```python
from build123d import *

# Parameters (mm, degrees)
CROQUIS1_W                 = 15
CROQUIS1_H                 = 13
SALIENTE_EXTRUIR1_DEPTH    = 3
REDONDEO1_R                = 3
CROQUIS6_R                 = 3
SALIENTE_EXTRUIR2_DEPTH    = 6
CORTAR_EXTRUIR1_DEPTH      = 66.261014396
CORTAR_EXTRUIR1_DEPTH_BACK = 66.261014396
CROQUIS2_R                 = 1.75
CORTAR_EXTRUIR2_DEPTH      = 63.24949799
CORTAR_EXTRUIR2_DEPTH_BACK = 63.24949799
CROQUIS3_R                 = 1.75
REDONDEO2_R                = 3


with BuildPart() as part:
    # Croquis1 → Saliente-Extruir1 (new, symmetric)
    with BuildSketch(Plane(origin=(0, 0, 0), x_dir=(1, 0, 0), z_dir=(0, 1, 0))):
        Polygon((0, 0), (0, 8), (14, 8), (14, 21), (0, 21), (0, 29), (55, 29), (55, 21), (41, 21), (41, 8), (55, 8), (55, 0), align=None)
        with Locations((27.5, 14.5)):
            Rectangle(CROQUIS1_W, CROQUIS1_H, mode=Mode.SUBTRACT)
    extrude(amount=SALIENTE_EXTRUIR1_DEPTH, both=True)

    # Redondeo1
    redondeo1_edges = [part.edges().sort_by_distance(p)[0] for p in [
        (0, -3, -4),
        (0, 3, -4),
        (0, -3, -25),
        (0, 3, -25),
        (55, -3, -4),
        (55, 3, -4),
        (55, 3, -25),
        (55, -3, -25),
    ]]
    fillet(redondeo1_edges, radius=REDONDEO1_R - 0.0001)  # a hair under: the kernel refuses the full size

    # Croquis6 → Saliente-Extruir2 (add)
    with BuildSketch(Plane.XY):
        with Locations(Location((3, 0, 0), (0, 0, 180))):
            Circle(CROQUIS6_R)
    extrude(amount=SALIENTE_EXTRUIR2_DEPTH)

    # Croquis2 → Cortar-Extruir1 (cut, two sides: drawn at the far end of the back side and taken through both)
    with BuildSketch(Plane.XY.offset(6).offset(-CORTAR_EXTRUIR1_DEPTH_BACK)):
        with Locations((3, 0)):
            Circle(CROQUIS2_R)
    extrude(amount=CORTAR_EXTRUIR1_DEPTH + CORTAR_EXTRUIR1_DEPTH_BACK, mode=Mode.SUBTRACT)

    # Croquis3 → Cortar-Extruir2 (cut, two sides: drawn at the far end of the back side and taken through both)
    with BuildSketch(Plane.XY.offset(-CORTAR_EXTRUIR2_DEPTH_BACK)):
        with Locations((52, 0)):
            Circle(CROQUIS3_R)
    extrude(amount=CORTAR_EXTRUIR2_DEPTH + CORTAR_EXTRUIR2_DEPTH_BACK, mode=Mode.SUBTRACT)

    # Redondeo2
    redondeo2_edges = [part.edges().sort_by_distance(p)[0] for p in [
        (14, 0, -8),
        (14, 0, -21),
        (41, 0, -21),
        (41, 0, -8),
        (20, 0, -21),
        (20, 0, -8),
        (35, 0, -8),
        (35, 0, -21),
    ]]
    fillet(redondeo2_edges, radius=REDONDEO2_R)


solid = part.part
```
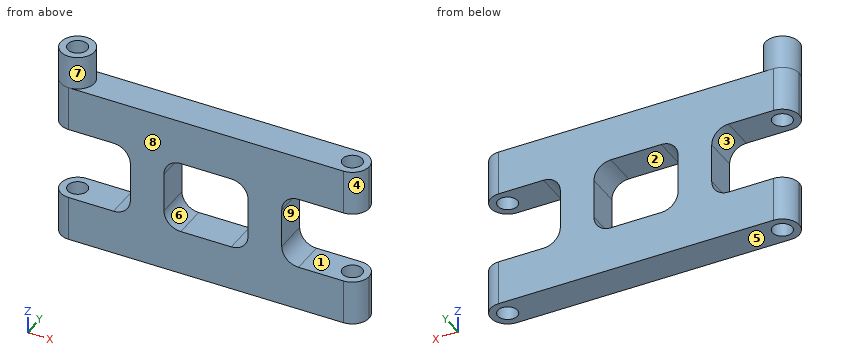
Verification items for the finished model (mm, model axes). Face numbers are marked on the shaded views. A direction names the side the tool comes from. Give positions to 0.01 mm unless a question says otherwise; leave off trailing zeros. Loops run counter-clockwise (first coordinate to the right, second up) from the corner with the lowest first, then second, coordinate; pieces in that order, holes last.
1. Go/stop test with flat-tipped pins: pin 1 Ø1.5 at (y, z) = (-1.5, -15.5) entering from -X; pin 2 Ø2 at (y, z) = (0.5, -19.5) entering from -X; pin 3 Ø3 at (y, z) = (-0.5, -16) entering from +X. Record where each tip stops, or that it passes through.
2. Thickness scan on line 1 (X direction, y = 0, z = -3); line 2 (Z direction, x = 8.5, y = 0.5); line 3 (Y direction, x = 52, z = -23). Record the ranges inside material, lowest first.
3. Section check A-A, the plane z = -9. Enter the section's corners in (x, y), then the cut area to 3 significant figures.
4. Set-up check for the marked faces 1, 2, 3, 4 and 5: record each of +Z, -Z, +X, -X, +Y, -Y from which the full face is reachable in a straight line by a thin tool's end or side.
5. Section check B-B, the plane x = 34. Enter the section's corners in (y, z).
6. Mould release check, pull along X, two halves, no side actions. Record for the marked faces 6, 7, 8 and 9: released by +X, released by -X, zero draft, split by the parting line, or undercut.
7. Section check C-C, the plane z = -25.5. Count the separate pieces of the cut face and the enclosed holes in it, then the cut area to 3 significant figures.
Geometry says:
1. pin 1: stops at x = 14
1. pin 2: stops at x = 12.66
1. pin 3: stops at x = 41
2. line 1: x = 0 to 1.25, 4.75 to 50.25, 53.75 to 55
2. line 2: z = -29 to -21, -8 to 0
2. line 3: y = -3 to -1.75, 1.75 to 3
3. outline: (13.24, -3) - (20.76, -3) - (20.76, 3) - (13.24, 3) - close; (34.24, -3) - (41.76, -3) - (41.76, 3) - (34.24, 3) - close
3. area: 90.3 mm2
4. face 1: +X, +Y, -Y
4. face 2: +Y, -Y
4. face 3: -X, +Y, -Y
4. face 4: +Z, -Z, +X, -Y
4. face 5: -Z, +X, -X, +Y, -Y
5. outline: (-3, -29) - (3, -29) - (3, -20.24) - (-3, -20.24) - close; (-3, -8.76) - (3, -8.76) - (3, 0) - (-3, 0) - close
6. face 6: undercut
6. face 7: split by the parting line
6. face 8: zero draft
6. face 9: released by +X
7. separate pieces: 1
7. enclosed holes: 2
7. area: 303 mm2
